Geometry check sheet. Reference: the model listing, model coordinates, mm. A direction names the side the tool comes from. Round coordinates to 2 decimals unless told otherwise and drop trailing zeros. Order: outer loops, then holes, each group sorted by start corner. A loop starts at its lowest first (then second) coordinate and runs counter-clockwise, first axis right, second up.
(1) Set-up check for faces 1 (the face through (0.616, -14.985, 0.66)), 2 (the face through (44.79, -1.86, 14.18)): record each of +Z, -Z, +X, -X, +Y, -Y from which the full face is reachable in a straight line by a thin tool's end or side.
(2) Go/stop test with flat-tipped pins: pin 1 (3 mm diameter, centred on x = -9, z = 4, fed in from -Y); pin 2 (4 mm diameter, centred on x = 5.5, z = 12, fed in from -Y). Record where each tip stops, or that it passes through.
(3) Sectioned sample at A-A (x = -27.5). Record the boundary of the cut face in (y, z), plus the area to 3 significant figures.
(4) Material ranges on line 1 along Z through (x, y) = (0, -0.75); line 2 along Z through (x, y) = (-39, -4.5); line 3 along Y through (x, z) = (-45, 0.5), recorded low to high.
(5) Release check for a two-part mould opening along X. For faces 3 (the face through (46.817, -14.985, 0.66)), 4 (the face through (49, 0, 0)), 5 (the face through (-44.79, -1.86, 14.18)) record: +X half, -X half, draft (parallel to the pull), parting line (faces both ways), or undercut.
from build123d import *

# Parameters (mm, degrees)
F0_R     = 15
F1_DEPTH = 49
F3_R     = 17.9592935662
F3_R_2   = 14.3
F4_DEPTH = 1.6
F5_SIZE  = 1


# Not quite as in the source:
# - a pattern or mirror of a feature is missing from the dataset's text; its kind, count and spacing are read off the source's solid


with BuildPart() as f1:
    # F0 (on Right) → F1 (new body, symmetric)
    with BuildSketch(Plane.YZ):
        Circle(F0_R)
    extrude(amount=F1_DEPTH, both=True)

    # F3 (on offset) → F4 (cut)
    with BuildSketch(Plane.YZ.offset(44)):
        Circle(F3_R)
        Circle(F3_R_2, mode=Mode.SUBTRACT)
    f4 = extrude(amount=F4_DEPTH, mode=Mode.SUBTRACT)

    # F4_copies: F4 across plane
    add(f4.mirror(Plane(origin=(0, 0, 0), x_dir=(0, 0, -1), z_dir=(-1, 0, 0))), mode=Mode.SUBTRACT)

    # F5
    f5_edges = [f1.edges().sort_by_distance(p)[0] for p in [
        (-49, -15, 0),
        (49, -15, 0),
    ]]
    chamfer(f5_edges, length=F5_SIZE)


solid = f1.part
Answer below:
1. face 1: +X, -X
1. face 2: none
2. pin 1: stops at y = -14.79
2. pin 2: stops at y = -11.18
3. outline: circle Ø30 at (0, 0)
3. area: 707 mm2
4. line 1: z = -14.98 to 14.98
4. line 2: z = -14.31 to 14.31
4. line 3: y = -14.29 to 14.29
5. face 3: draft
5. face 4: +X half
5. face 5: undercut
